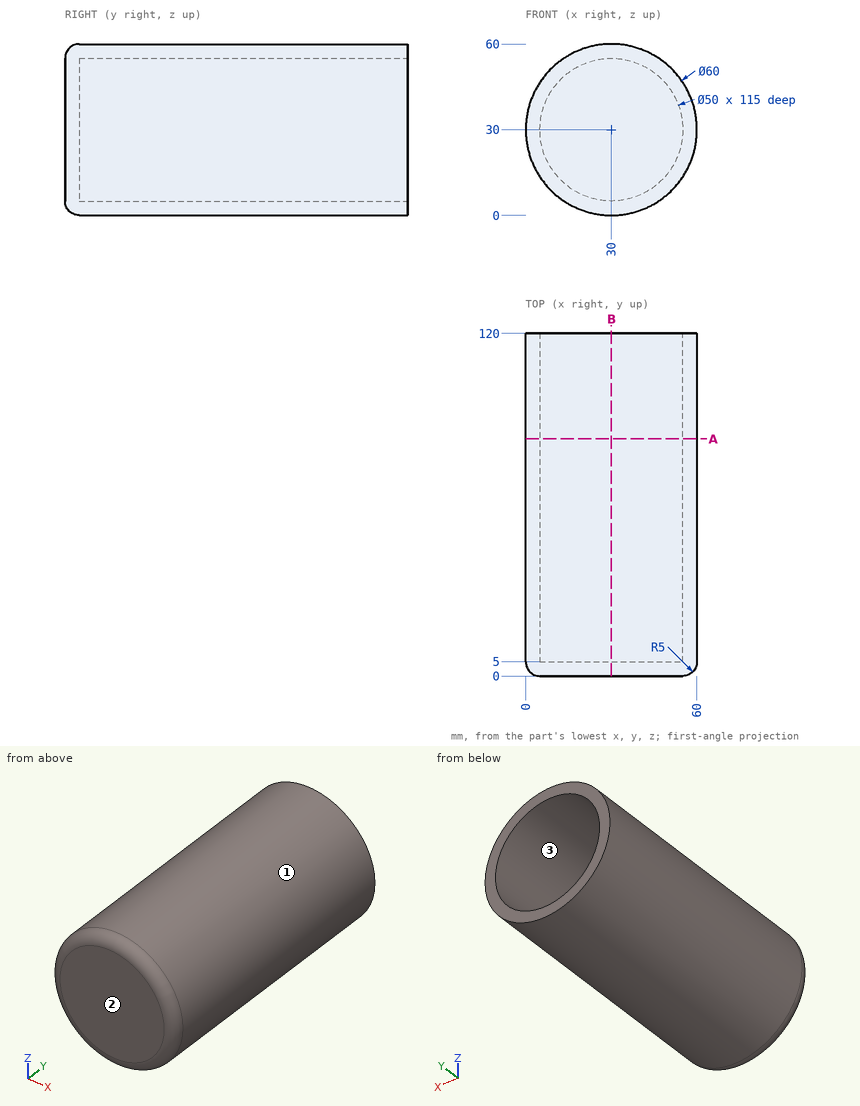
Print and shaded views of the part. All mm, measured from the part's lowest x, y and z. Coordinates: 2 decimals unless noted, no trailing zeros. Order: outer loops, then holes, each group sorted by start corner. A loop starts at its lowest first (then second) coordinate and runs counter-clockwise, first axis right, second up. Notation, with made-up numbers: (-27, 31.5) - (-7, 31.5) arc R17 ccw to (-7, 51.5) - close; hole circle Ø9 at (22, 79). An arc over 180 degrees is marked (long way). Put each result on its own line as item: value.
1. Saw through at B-B (x = 30). Write the cut outline in (y, z), and give its area (3 significant figures).
Answer sheet:
outline: (0, 5) arc R5 ccw to (5, 0) - (120, 0) - (120, 5) - (5, 5) - (5, 55) - (120, 55) - (120, 60) - (5, 60) arc R5 ccw to (0, 55) - close
area: 1,440 mm^2
2. Pull direction X, two halves, no side cores. Call the marked faces 1, 2 and 3: pulls with the +X half, pulls with the -X half, needs draft (parallel to the pull), parting line crosses it, or undercut.
Answer sheet:
face 1: parting line crosses it
face 2: needs draft
face 3: undercut
3. Saw through at A-A (y = 83). Write the cut outline in (x, z).
Answer sheet:
outline: circle Ø60 at (30, 30); hole circle Ø50 at (30, 30)
4. Probe line 1 along Z through (x, y) = (30, 77); line 2 along X through (y, z) = (42.5, 31); line 3 along Y through (x, z) = (24, 11). List the from-to ranges inside material, lowest first. Write a range as [from, to].
Answer sheet:
line 1: z = [0, 5], [55, 60]
line 2: x = [0.02, 5.02], [54.98, 59.98]
line 3: y = [0, 5]
5. Drop flat-ended pins along their axis: P1, Ø10, axis at y = 99, z = 20, coming from the +X side; P2, Ø15, axis at x = 21, z = 17.5, coming from the +Y side; P3, Ø12, axis at y = 64, z = 54, coming from the -X side. Give the stop position or say it passes through.
Answer sheet:
P1: stops at x = 59.58
P2: stops at y = 5
P3: stops at x = 6
